from build123d import *


with BuildPart() as part:
    # Sketch1 → Revolve1 (revolve)
    with BuildSketch(Plane.XY):
        with BuildLine():
            Line((180.862254067, -468.383325669), (171.360424036, -468.383325669))
            ThreePointArc((171.360424036, -468.383325669), (174.804519989, -467.007991593), (176.353902933, -463.638606894))
            Line((176.353902933, -463.638606894), (206.516426137, 126.361393106))
            ThreePointArc((206.516426137, 126.361393106), (205.147613164, 130.060770285), (201.52294724, 131.616674331))
            Line((201.52294724, 131.616674331), (200.860485156, 131.616674331))
            Line((200.860485156, 131.616674331), (170.983852863, -452.791099984))
            ThreePointArc((170.983852863, -452.791099984), (169.434469919, -456.160484683), (165.990373966, -457.535818758))
            Line((165.990373966, -457.535818758), (-149.139514844, -457.535818758))
            Line((-149.139514844, -457.535818758), (-149.139514844, -487.535818758))
            Line((-149.139514844, -487.535818758), (187.943679345, -487.535818758))
            ThreePointArc((187.943679345, -487.535818758), (192.563077007, -484.44923592), (191.479213251, -479.000284853))
            Line((191.479213251, -479.000284853), (180.862254067, -468.383325669))
        make_face()
    revolve(axis=Axis((-150.008312882, -212.837137396, 0), (0, -1, 0)))


solid = part.part
Read the model definition and answer for the solid it produces. Units are mm, in the model's axes. A direction names the side the tool comes from. Round coordinates to 2 decimals unless told otherwise and drop trailing zeros. Write each loop counter-clockwise with the first axis right and the second up, starting at its lowest first coordinate (ties: lowest second). Pieces come first, ordered by that corner, then holes.
1. The part is cut by section A-A, the plane y = 32. Determine the outline of the cut face in (x, z), then the cut area to 3 significant figures.
2. The part is cut by section B-B, the plane y = -326.5. Determine the outline of the cut face in (x, z), then the cut area to 3 significant figures.
3. Straight lines are drawn through the part: L1, parallel to Y at x = 94.5, z = 58.5; L2, parallel to X at y = -247, z = -148; L3, parallel to X at y = -151, z = -283. For each, find the intervals that lie inside material, in ascending order.
4. Which of the six approach directions +Z, -Z, +X, -X, +Y, -Y give full straight-line access (tool end or side, diameter ignored) to faces 1 (the face through (170.21, -164.68, 100.84)), 2 (the face through (-194.485, -164.509, 338.747))?
5. Determine the mould class of faces 3 (the face through (-154, -457.536, 4)), 4 (the face through (-412.985, -468.899, -201.643)), 5 (the face through (-145, -487.536, 5)) for opening direction X: pulls with the +X half, pulls with the -X half, needs draft (parallel to the pull), parting line crosses it, or undercut.
6. Given pin 1 Ø3 at (y, z) = (-421.5, 278.5) entering from +X; pin 2 Ø12 at (x, z) = (-94, -71) entering from +Y; pin 3 Ø3 at (y, z) = (15.5, 107) entering from +X, each flat-ended and moving along its own axis, determine where each tip first touches the part or whether it passes through.
Values:
1. outline: circle Ø703.4 at (-150.01, 0); hole circle Ø691.55 at (-150.01, 0)
1. area: 13,000 mm2
2. outline: circle Ø666.75 at (-150.01, 0); hole circle Ø654.9 at (-150.01, 0)
2. area: 12,300 mm2
3. L1: y = -487.54 to -457.54
3. L2: x = -453.26 to -446.65, 146.63 to 153.24
3. L3: x = -342.65 to -331.91, 31.9 to 42.63
4. face 1: +Y
4. face 2: none
5. face 3: undercut
5. face 4: parting line crosses it
5. face 5: needs draft
6. pin 1: stops at x = 26.61
6. pin 2: stops at y = -457.54
6. pin 3: stops at x = 184.62
